Check sheet for the modelled part. Datum: model origin and axes. Units: mm. Face numbers are marked on the shaded views. A direction names the side the tool comes from. Give positions to 0.01 mm unless a question says otherwise; leave off trailing zeros. Write each loop counter-clockwise with the first axis right and the second up, starting at its lowest first coordinate (ties: lowest second). Pieces come first, ordered by that corner, then holes. Notation, with made-up numbers: (-36, 65.5) -> (-25, 65.5) arc R7 ccw to (-25, 75.5) -> close; hole circle Ø10 at (-8.75, 53.5). An arc over 180 degrees is marked (long way). Answer as a JSON object with one key per item and string values.
from build123d import *

# Parameters (mm, degrees)
F1_DEPTH = 2
F0_R     = 1.3
F0_R_2   = 1.5
F2_DEPTH = 4
F3_DEPTH = 6
F0_W     = 41.5
F0_H     = 53.6
F4_DEPTH = 7
F0_W_2   = 44.5
F0_H_2   = 56.6
F5_DEPTH = 6
F6_W     = 30.5
F6_H     = 1.5
F7_DEPTH = 3


# Not quite as in the source:
# - a fillet or chamfer that OpenCascade refuses, or shapes differently, is made with other operations: its cross-section is extruded or revolved along the edge and cut away or added
# - a feature names something its author has since deleted; it is built from what else it names


with BuildPart() as f1:
    # F0 (on Top) → F1 (new body)
    with BuildSketch(Plane.XY):
        with BuildLine():
            ThreePointArc((0, 5.75), (5.2603266711, 5.2603266711), (5.75, 0))
            Line((5.75, 0), (32.75, 0))
            ThreePointArc((32.75, 0), (33.3948928082, 5.1051071918), (38.5, 5.75))
            Line((38.5, 5.75), (38.5, 44.1))
            ThreePointArc((38.5, 44.1), (33.4963752154, 45.5963752154), (32, 50.6))
            Line((32, 50.6), (6.5, 50.6))
            ThreePointArc((6.5, 50.6), (5.1593928501, 45.4406071499), (0, 44.1))
            Line((0, 44.1), (0, 5.75))
        make_face()
    extrude(amount=F1_DEPTH)

    # F0 (on Top) → F2 (join)
    with BuildSketch(Plane.XY):
        with BuildLine():
            Line((0, 50.6), (0, 44.1))
            ThreePointArc((0, 44.1), (5.1593928501, 45.4406071499), (6.5, 50.6))
            Line((6.5, 50.6), (0, 50.6))
        make_face()
        with Locations((3.05, 47.3)):
            Circle(F0_R, mode=Mode.SUBTRACT)
        with BuildLine():
            ThreePointArc((32, 50.6), (33.4963752154, 45.5963752154), (38.5, 44.1))
            Line((38.5, 44.1), (38.5, 50.6))
            Line((38.5, 50.6), (32, 50.6))
        make_face()
        with Locations((35.8, 47.3)):
            Circle(F0_R, mode=Mode.SUBTRACT)
        with BuildLine():
            ThreePointArc((38.5, 5.75), (33.3948928082, 5.1051071918), (32.75, 0))
            Line((32.75, 0), (38.5, 0))
            Line((38.5, 0), (38.5, 5.75))
        make_face()
        with Locations((35.44, 2.9)):
            Circle(F0_R_2, mode=Mode.SUBTRACT)
        with BuildLine():
            Line((0, 5.75), (0, 0))
            Line((0, 0), (5.75, 0))
            ThreePointArc((5.75, 0), (5.2603266711, 5.2603266711), (0, 5.75))
        make_face()
        with Locations((3.01, 3.25)):
            Circle(F0_R_2, mode=Mode.SUBTRACT)
    extrude(amount=F2_DEPTH)

    # F0 (on Top) → F3 (join)
    with BuildSketch(Plane.XY):
        with Locations((3.05, 47.3)):
            Circle(F0_R)
        with Locations((35.8, 47.3)):
            Circle(F0_R)
    extrude(amount=F3_DEPTH)

    # F0 (on Top) → F4 (join)
    with BuildSketch(Plane.XY):
        with Locations((19.25, 25.3)):
            Rectangle(F0_W, F0_H)
        Polygon((5.75, 0), (0, 0), (0, 5.75), (0, 44.1), (0, 50.6), (6.5, 50.6), (32, 50.6), (38.5, 50.6), (38.5, 44.1), (38.5, 5.75), (38.5, 0), (32.75, 0), align=None, mode=Mode.SUBTRACT)
    extrude(amount=F4_DEPTH)

    # F0 (on Top) → F5 (join)
    with BuildSketch(Plane.XY):
        with Locations((19.25, 25.3)):
            Rectangle(F0_W_2, F0_H_2)
        with Locations((19.25, 25.3)):
            Rectangle(F0_W, F0_H, mode=Mode.SUBTRACT)
    extrude(amount=F5_DEPTH)

    # F6 (on face) → F7 (cut)
    with BuildSketch(Plane(origin=(0, 53.6, 0), x_dir=(-1, 0, 0), z_dir=(0, 1, 0))):
        with Locations((-19.25, 6.25)):
            Rectangle(F6_W, F6_H)
    extrude(amount=-F7_DEPTH, mode=Mode.SUBTRACT)

    # F8: chamfer of 0.4 x 2.0578216064 on 2 edges, made by hand


with BuildPart() as f8_tool2:
    # F8_s3 → F8_t4 (revolve)
    with BuildSketch(Plane.XZ.offset(-47.3)):
        Polygon((37.1, 3.9421783936), (36.7, 6), (37.1, 6), align=None)
    revolve(axis=Axis((35.8, 47.3, 6), (0, 0, 1)))

    split(bisect_by=Plane.XY.offset(4), keep=Keep.TOP)


with BuildPart() as f1_1:
    add(f1.part)

    # F8_t1: cut F8_tool2
    add(f8_tool2.part, mode=Mode.SUBTRACT)


with BuildPart() as f8_tool7:
    # F8_s8 → F8_t9 (revolve)
    with BuildSketch(Plane.XZ.offset(-47.3)):
        Polygon((4.35, 3.9421783936), (3.95, 6), (4.35, 6), align=None)
    revolve(axis=Axis((3.05, 47.3, 6), (0, 0, 1)))

    split(bisect_by=Plane.XY.offset(4), keep=Keep.TOP)


with BuildPart() as f1_2:
    add(f1_1.part)

    # F8_t6: cut F8_tool7
    add(f8_tool7.part, mode=Mode.SUBTRACT)


solid = f1_2.part
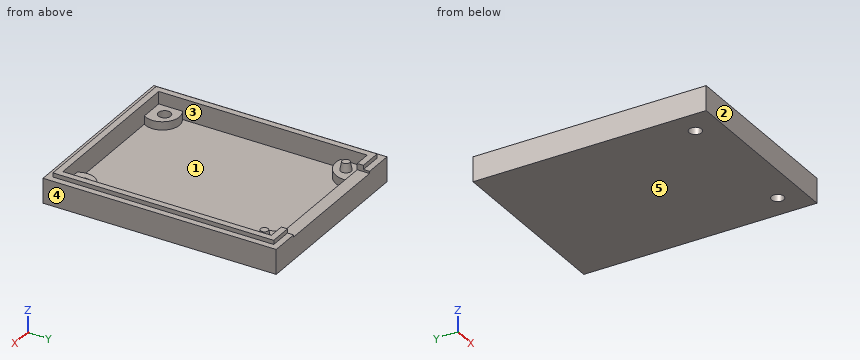
1. Scan lines: L1, parallel to X at y = 26.5, z = 3.25; L2, parallel to Y at x = 4.5, z = 5.25; L3, parallel to Y at x = 35.44, z = 2.3. Record each from-to range of solid material in increasing order. Write a range as [from, to].
Determined:
{"L1": "[-3, 0], [38.5, 41.5]", "L2": "[-3, 0], [50.6, 53.6]", "L3": "[-3, 1.4], [4.4, 6.23], [44.34, 53.6]"}
2. Sectioned sample at A-A, the plane x = 3.05. Enter the section's corners in (y, z).
Determined:
{"outline": "(-3, 0) -> (1.75, 0) -> (1.75, 4) -> (0, 4) -> (0, 7) -> (-1.5, 7) -> (-1.5, 6) -> (-3, 6) -> close; (4.75, 0) -> (53.6, 0) -> (53.6, 6) -> (52.1, 6) -> (52.1, 7) -> (50.6, 7) -> (50.6, 4) -> (48.59, 4) -> (48.2, 6) -> (46.4, 6) -> (46.01, 4) -> (44.15, 4) -> (44.15, 2) -> (6.41, 2) -> (6.41, 4) -> (4.75, 4) -> close"}
3. Go/stop test with flat-tipped pins: P1, Ø0.5, axis at x = 0.5, z = 6.5, coming from the +Y side; P2, Ø0.5, axis at x = 36, y = 47, coming from the +Z side; P3, Ø0.9, axis at x = 21, y = 52.5, coming from the +Z side. Record where each tip stops, or that it passes through.
Determined:
{"P1": "y = 52.1", "P2": "z = 6", "P3": "z = 5.5"}
4. Sectioned sample at B-B, the plane x = 25.5. Enter the section's corners in (y, z), plus the area to 3 significant figures.
Determined:
{"outline": "(-3, 0) -> (53.6, 0) -> (53.6, 5.5) -> (50.6, 5.5) -> (50.6, 2) -> (0, 2) -> (0, 7) -> (-1.5, 7) -> (-1.5, 6) -> (-3, 6) -> close", "area": "137 mm^2"}
5. Access from +Z, -Z, +X, -X, +Y, -Y to the whole of each face (thin tool, end or side, straight path). Record for the marked faces 1 and 2.
Determined:
{"face 1": "+Z", "face 2": "+Z, -Z, +X, -X, -Y"}
6. Sectioned sample at D-D, the plane x = 35.8. Enter the section's corners in (y, z), plus the area to 3 significant figures.
Determined:
{"outline": "(-3, 0) -> (1.44, 0) -> (1.44, 4) -> (0, 4) -> (0, 7) -> (-1.5, 7) -> (-1.5, 6) -> (-3, 6) -> close; (4.36, 0) -> (53.6, 0) -> (53.6, 6) -> (52.1, 6) -> (52.1, 7) -> (50.6, 7) -> (50.6, 4) -> (48.59, 4) -> (48.2, 6) -> (46.4, 6) -> (46.01, 4) -> (44.22, 4) -> (44.22, 2) -> (6.3, 2) -> (6.3, 4) -> (4.36, 4) -> close", "area": "158 mm^2"}
7. Mould release check, pull along X, two halves, no side actions. Record for the marked faces 3, 4 and 5: released by +X, released by -X, zero draft, split by the parting line, or undercut.
Determined:
{"face 3": "undercut", "face 4": "released by +X", "face 5": "zero draft"}
8. Sectioned sample at C-C, the plane y = 41.5. Enter the section's corners in (x, z), plus the area to 3 significant figures.
Determined:
{"outline": "(-3, 0) -> (41.5, 0) -> (41.5, 6) -> (40, 6) -> (40, 7) -> (38.5, 7) -> (38.5, 2) -> (0, 2) -> (0, 7) -> (-1.5, 7) -> (-1.5, 6) -> (-3, 6) -> close", "area": "116 mm^2"}
